```python
from build123d import *

# Parameters (mm, degrees)
F0_R      = 66.2686
F0_R_2    = 63.5
F1_DEPTH  = 406.4
F3_DEPTH  = 66.2696
F5_DEPTH  = 9.525
F6_W      = 152.4
F6_H      = 152.5488182802
F6_W_2    = 139.7
F6_H_2    = 139.8488182802
F7_DEPTH  = 9.525
F8_W      = 152.4
F8_H      = 152.5488182802
F9_DEPTH  = 9.525
F10_DEPTH = 28.576
F11_W     = 139.7
F11_H     = 9.525
F12_DEPTH = 25.4


with BuildPart() as f1:
    # F0 (on Top) → F1 (new body)
    with BuildSketch(Plane.XY):
        Circle(F0_R)
        Circle(F0_R_2, mode=Mode.SUBTRACT)
    extrude(amount=F1_DEPTH)

    # F2 (on Front) → F3 (cut, through all)
    with BuildSketch(Plane.XZ):
        with BuildLine():
            Line((-12.7, 203.2), (-12.7, 101.6))
            ThreePointArc((-12.7, 101.6), (-8.9802561211, 92.6197438789), (0, 88.9))
            ThreePointArc((0, 88.9), (8.9802561211, 92.6197438789), (12.7, 101.6))
            Line((12.7, 101.6), (12.7, 203.2))
            Line((12.7, 203.2), (12.7, 304.8))
            ThreePointArc((12.7, 304.8), (0, 317.5), (-12.7, 304.8))
            Line((-12.7, 304.8), (-12.7, 203.2))
        make_face()
    extrude(amount=-F3_DEPTH, mode=Mode.SUBTRACT)

    # F4 (on Top) → F5 (join)
    with BuildSketch(Plane.XY):
        Polygon((-76.2, 76.2159317421), (-76.2, 0.0159317421), (-76.2, -76.3328865381), (76.2, -76.3328865381), (76.2, 76.2159317421), align=None)
    extrude(amount=-F5_DEPTH)

    # F6 (on face) → F7 (join)
    with BuildSketch(Plane(origin=(0, 0, -9.525), x_dir=(1, 0, 0), z_dir=(0, 0, -1))):
        with Locations((0, 0.058477398)):
            Rectangle(F6_W, F6_H)
        with Locations((0, 0.058477398)):
            Rectangle(F6_W_2, F6_H_2, mode=Mode.SUBTRACT)
    extrude(amount=F7_DEPTH)

    # F8 (on face) → F9 (join)
    with BuildSketch(Plane(origin=(0, 0, -19.05), x_dir=(1, 0, 0), z_dir=(0, 0, -1))):
        with Locations((0, 0.058477398)):
            Rectangle(F8_W, F8_H)
    extrude(amount=F9_DEPTH)

    # F10 (cut, through all): a face of the model
    f10_faces = [f1.faces().sort_by_distance(p)[0] for p in [
        (0, 0, 0),
    ]]
    extrude(f10_faces, amount=-F10_DEPTH, mode=Mode.SUBTRACT)

    # F11 (on face) → F12 (cut)
    with BuildSketch(Plane.YZ.offset(76.2)):
        with Locations((-0.1328865381, -14.2875)):
            Rectangle(F11_W, F11_H)
    extrude(amount=-F12_DEPTH, mode=Mode.SUBTRACT)


solid = f1.part
```
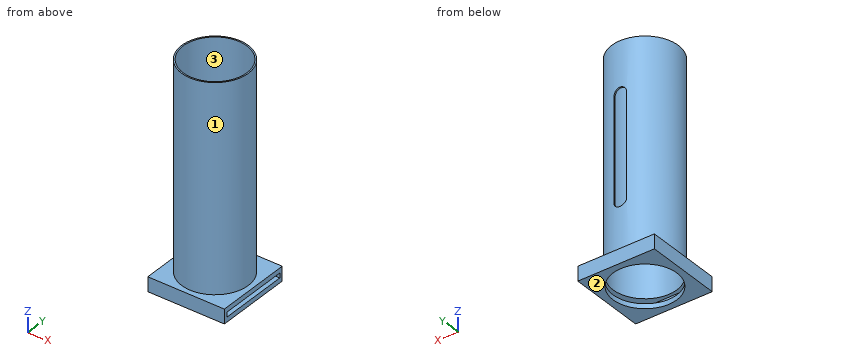
Work out the finished part from the listing and answer in its coordinate system (mm). Face numbers are marked on the shaded views. Give positions to 0.01 mm unless a question says otherwise; leave off trailing zeros. Order: outer loops, then holes, each group sorted by start corner. A loop starts at its lowest first (then second) coordinate and runs counter-clockwise, first axis right, second up. Notation, with made-up numbers: (32.25, 43) -> (84.25, 43) arc R21 ccw to (84.25, 54) -> close; hole circle Ø11 at (87.25, 81). An arc over 180 degrees is marked (long way). Answer as CSV lines item,"result". Start each with the question number.
(1) Section A-A, the plane y = 0 is taken. Write down the section's boundary in (x, z) (3 decimals), plus the area to 3 significant figures.
(2) Section B-B, the plane x = 38.5 is taken. Write down the section's boundary in (y, z) (3 decimals).
(3) Section D-D, the plane y = -36 is taken. Write down the section's boundary in (x, z) (3 decimals).
(4) Each of these flat-tipped pins is pushed along its axis until it touches: pin 1 Ø12 at (y, z) = (47.5, 74) entering from +X; pin 2 Ø1.5 at (x, z) = (27.5, 279) entering from -Y; pin 3 Ø10.5 at (y, z) = (-11, -15) entering from +X; pin 4 Ø6 at (y, z) = (-54.5, 137.5) entering from -X. Where does it stop, or does it pass through?
(5) For a pull along X with two mould halves and no side action, classify the marked faces 1, 2 and 3 as released by +X, released by -X, zero draft, split by the parting line, or undercut.
(6) Consider line 1 along Y through (x, z) = (0, -23.5); line 2 along Z through (x, y) = (-66, 7.5) (3 decimals); line 3 along X through (y, z) = (-18.5, 243.5). Determine where each line is inside the solid, lowest interval first.
(7) Section C-C, the plane z = 9 is taken. Write down the section's boundary in (x, y).
Entries:
1,outline,"(-76.2, -28.575) -> (-63.5, -28.575) -> (-63.5, -19.05) -> (-69.85, -19.05) -> (-69.85, -9.525) -> (-63.5, -9.525) -> (-63.5, 406.4) -> (-66.269, 406.4) -> (-66.269, 0) -> (-76.2, 0) -> close; (63.5, -28.575) -> (76.2, -28.575) -> (76.2, -19.05) -> (63.5, -19.05) -> close; (63.5, -9.525) -> (76.2, -9.525) -> (76.2, 0) -> (66.269, 0) -> (66.269, 406.4) -> (63.5, 406.4) -> close"
1,area,"2,790 mm²"
2,outline,"(-76.333, -28.575) -> (-50.498, -28.575) -> (-50.498, -19.05) -> (-69.983, -19.05) -> (-69.983, -9.525) -> (-50.498, -9.525) -> (-50.498, 406.4) -> (-53.938, 406.4) -> (-53.938, 0) -> (-76.333, 0) -> close; (50.498, -28.575) -> (76.216, -28.575) -> (76.216, 0) -> (53.938, 0) -> (53.938, 406.4) -> (50.498, 406.4) -> (50.498, -9.525) -> (69.866, -9.525) -> (69.866, -19.05) -> (50.498, -19.05) -> close"
3,outline,"(-76.2, -28.575) -> (-52.309, -28.575) -> (-52.309, -19.05) -> (-69.85, -19.05) -> (-69.85, -9.525) -> (-52.309, -9.525) -> (-52.309, 406.4) -> (-55.637, 406.4) -> (-55.637, 0) -> (-76.2, 0) -> close; (52.309, -28.575) -> (76.2, -28.575) -> (76.2, -19.05) -> (52.309, -19.05) -> close; (52.309, -9.525) -> (76.2, -9.525) -> (76.2, 0) -> (55.637, 0) -> (55.637, 406.4) -> (52.309, 406.4) -> close"
4,pin 1,"x = 51.67"
4,pin 2,"y = -60.63"
4,pin 3,"x = 76.2"
4,pin 4,"x = -41.7"
5,face 1,"split by the parting line"
5,face 2,"zero draft"
5,face 3,"undercut"
6,line 1,"-76.33 to -63.5, 63.5 to 76.22"
6,line 2,"-28.575 to -19.05, -9.525 to 0"
6,line 3,"-63.63 to -60.75, 60.75 to 63.63"
7,outline,"circle Ø132.54 at (0, 0); hole circle Ø127 at (0, 0)"
